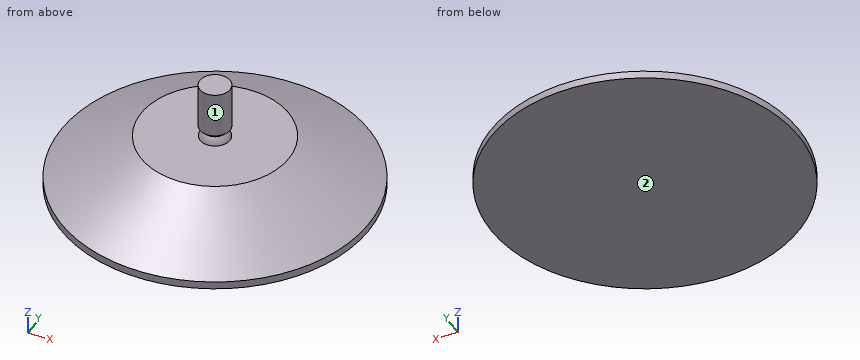
from build123d import *

# Parameters (mm, degrees)
ESQUISSE1_R        = 40
BOSS_EXTRU_1_DEPTH = 2
ESQUISSE2_R        = 40
BOSS_EXTRU_2_DEPTH = 12
BOSS_EXTRU_2_TAPER = 60


with BuildPart() as part:
    # Esquisse1 → Boss.-Extru.1 (new body)
    with BuildSketch(Plane.XY):
        Circle(ESQUISSE1_R)
    extrude(amount=BOSS_EXTRU_1_DEPTH)

    # Esquisse2 → Boss.-Extru.2 (add)
    with BuildSketch(Plane.XY.offset(2)):
        Circle(ESQUISSE2_R)
    extrude(amount=BOSS_EXTRU_2_DEPTH, taper=BOSS_EXTRU_2_TAPER)

    # Esquisse3 → Révolution1 (revolve)
    with BuildSketch(Plane(origin=(0, 0, 0), x_dir=(1, 0, 0), z_dir=(0, 1, 0))):
        with BuildLine():
            Line((2.828427125, -15.907299026), (3.932041335, -17.010913236))
            Line((3.932041335, -17.010913236), (3.932041335, -28.955760853))
            Line((3.932041335, -28.955760853), (0, -28.955760853))
            Line((0, -28.955760853), (0, -9.078871902))
            ThreePointArc((0, -9.078871902), (3.69551813, -11.548138172), (2.828427125, -15.907299026))
        make_face()
    revolve(axis=Axis((0, 0, 28.955760853), (0, 0, -1)))


solid = part.part
Can you work these out from the model? Positions are in its coordinate system, mm. Face numbers are marked on the shaded views. A direction names the side the tool comes from. Coordinates: 2 decimals unless noted, no trailing zeros. Write each loop counter-clockwise with the first axis right and the second up, starting at its lowest first coordinate (ties: lowest second). Pieces come first, ordered by that corner, then holes. Notation, with made-up numbers: (52, 7.25) -> (100, 7.25) arc R32 ccw to (100, 37.25) -> close; hole circle Ø5 at (82, 36.5). An arc over 180 degrees is marked (long way). Write each question's results on one line, items separated by ' | '. Start each with the question number.
Q1. Imagine slicing it at D-D (z = 7.75). Write out the boundary of the cut face in (x, y), then the cut area to 3 significant figures.
Q2. Imagine slicing it at C-C (z = 21.5). Write out the boundary of the cut face in (x, y), then the cut area to 3 significant figures.
Q3. If I drill on probe 1 along Z at (x, y) = (-10, -5); probe 2 along X at (y, z) = (17, 8.5); probe 3 along Z at (x, y) = (23, 21.5), over which ranges is the centre line in solid material (lowest first)?
Q4. I'm going to push flat-ended pins straight in: pin 1 (3 mm diameter, centred on x = -14, z = 10.5, fed in from -Y); pin 2 (4 mm diameter, centred on x = 6.5, y = 10, fed in from +Z); pin 3 (4 mm diameter, centred on y = -17, z = 3.5, fed in from -X); pin 4 (1.5 mm diameter, centred on y = -7.5, z = 15, fed in from -X). Where does each tip first touch, or does it pass through?
Q5. Imagine slicing it at A-A (y = 0). Write out the boundary of the cut face in (x, z), then the cut area to 3 significant figures.
Q6. On a 3-axis mill with a long thin cutter (end or side, diameter ignored), from which of +Z, -Z, +X, -X, +Y, -Y can I reach the whole of each face in a straight line? I mean the marked faces 1 and 2. Say none if no direction works.
Taken from the geometry:
1) outline: circle Ø60.08 at (0, 0) | area: 2,840 mm^2
2) outline: circle Ø7.86 at (0, 0) | area: 48.6 mm^2
3) probe 1: z = 0 to 14 | probe 2: x = -23.18 to 23.18 | probe 3: z = 0 to 6.92
4) pin 1: stops at y = -24.23 | pin 2: stops at z = 14 | pin 3: stops at x = -36.8 | pin 4: passes through
5) outline: (-40, 0) -> (40, 0) -> (40, 2) -> (19.22, 14) -> (3.89, 14) arc R4 ccw to (2.83, 15.91) -> (3.93, 17.01) -> (3.93, 28.96) -> (-3.93, 28.96) -> (-3.93, 17.01) -> (-2.83, 15.91) arc R4 ccw to (-3.89, 14) -> (-19.22, 14) -> (-40, 2) -> close | area: 985 mm^2
6) face 1: +Z | face 2: -Z, +X, -X, +Y, -Y
